Work out the finished part from the listing and answer in its coordinate system (mm). A direction names the side the tool comes from. Coordinates: 2 decimals unless noted, no trailing zeros. Write each loop counter-clockwise with the first axis right and the second up, starting at its lowest first coordinate (ties: lowest second). Pieces come first, ordered by that corner, then holes. Notation, with made-up numbers: (15, -3) - (48, -3) arc R28 cw to (48, 30) - close; hole circle Ø5 at (3.5, -11). An arc over 180 degrees is marked (long way). Use one line per item in the form item = value. Start each with the question number.
Item 1: Consider probe 1 along X at (y, z) = (0, -28); probe 2 along X at (y, z) = (-9, -29); probe 3 along Z at (x, y) = (4.5, 16). Determine where each line is inside the solid, lowest interval first.
Item 2: Given pin 1 (1 mm diameter, centred on y = -13.5, z = -20.5, fed in from +X); pin 2 (3 mm diameter, centred on x = 0.5, z = -20.5, fed in from +Y); pin 3 (1.5 mm diameter, centred on y = -10, z = -23.5, fed in from +X), each flat-ended and moving along its own axis, determine where each tip first touches the part or whether it passes through.
Item 3: A cutting plane is placed at A-A (z = -23). Write down the section's boundary in (x, y).
Item 4: For faces 4 (the flat face through (0, 14, -15)), 5 (the flat face through (-15, 0, 2.5)), determine the directions among +Z, -Z, +X, -X, +Y, -Y from which every point of the face is accessible in a straight line to the end or side of a thin tool.
Item 5: Determine the mould class of faces 1 (the flat face through (-9, 12, 0)), 2 (the cylindrical face through (-0.372, -19.997, 0.246)), 3 (the flat face through (-1, 14, -15)) for opening direction X: released by +X, released by -X, zero draft, split by the parting line, or undercut.
from build123d import *

# Parameters (mm, degrees)
F0_R     = 14.7
F0_R_2   = 13.45
F1_DEPTH = 38.1
F0_R_3   = 20
F2_DEPTH = 2.5
F3_SIZE  = 2
F4_R     = 1
F5_W     = 26.7045460641
F5_H     = 56.1363650486
F6_DEPTH = 1


with BuildPart() as f1:
    # F0 (on Top) → F1 (new body)
    with BuildSketch(Plane.XY):
        Circle(F0_R)
        Circle(F0_R_2, mode=Mode.SUBTRACT)
    extrude(amount=-F1_DEPTH)

    # F0 (on Top) → F2 (join)
    with BuildSketch(Plane.XY):
        Circle(F0_R_3)
        Circle(F0_R, mode=Mode.SUBTRACT)
        Circle(F0_R)
        Circle(F0_R_2, mode=Mode.SUBTRACT)
    extrude(amount=F2_DEPTH)

    # F3
    f3_edges = [f1.edges().sort_by_distance(p)[0] for p in [
        (-20, 0, 2.5),
    ]]
    chamfer(f3_edges, length=F3_SIZE)

    # F4
    f4_edges = [f1.edges().sort_by_distance(p)[0] for p in [
        (-13.45, 0, 2.5),
    ]]
    fillet(f4_edges, radius=F4_R)

    # F5 (on Right) → F6 (cut)
    with BuildSketch(Plane.YZ):
        with Locations((13.3522730321, -17.5000005402)):
            Rectangle(F5_W, F5_H)
    extrude(amount=-F6_DEPTH, mode=Mode.SUBTRACT)


solid = f1.part
Answer:
q1.probe_1 = -14.7 to -13.45, 13.45 to 14.7
q1.probe_2 = -11.62 to -10, 10 to 11.62
q1.probe_3 = 0 to 2.5
q2.pin_1 = 6.86
q2.pin_2 = 14.7
q2.pin_3 = 11.42
q3.outline = (-1, 13.41) - (-1, 14.67) arc R14.7 ccw (long way) to (0, 14.7) - (0, 13.45) arc R13.45 cw (long way) to start
q4.face_4 = +Z, -Z, +Y
q4.face_5 = +Z, +X, -X, +Y, -Y
q5.face_1 = zero draft
q5.face_2 = split by the parting line
q5.face_3 = undercut
